from build123d import *

# Parameters (mm, degrees)
SKETCH1_R      = 3.378193244
EXTRUDE1_DEPTH = 300


with BuildPart() as part:
    # Sketch1 → Extrude1 (new body)
    with BuildSketch(Plane.XY):
        with BuildLine():
            Line((-17.04042372, 15.431408639), (-24.485570149, 7.990664768))
            ThreePointArc((-24.485570149, 7.990664768), (-25.653755155, 5.34518984), (-24.733349861, 2.603648687))
            ThreePointArc((-24.733349861, 2.603648687), (-18.529607307, -7.672004621), (-15.653778055, -19.325548231))
            ThreePointArc((-15.653778055, -19.325548231), (-14.366806417, -21.915316136), (-11.67045068, -22.960715361))
            Line((-11.67045068, -22.960715361), (-1.144536244, -22.960715361))
            ThreePointArc((-1.144536244, -22.960715361), (-0.031123661, -22.499524769), (0.430066931, -21.386112187))
            Line((0.430066931, -21.386112187), (0.430066931, -20.471826472))
            ThreePointArc((0.430066931, -20.471826472), (-0.031123661, -19.35841389), (-1.144536244, -18.897223298))
            Line((-1.144536244, -18.897223298), (-1.851013704, -18.897223298))
            ThreePointArc((-1.851013704, -18.897223298), (-2.114950893, -19.003860844), (-2.230734754, -19.263915653))
            Line((-2.230734754, -19.263915653), (-2.231730696, -19.292435705))
            ThreePointArc((-2.231730696, -19.292435705), (-2.347514556, -19.552490514), (-2.611451745, -19.65912806))
            Line((-2.611451745, -19.65912806), (-4.522314022, -19.65912806))
            ThreePointArc((-4.522314022, -19.65912806), (-5.420227395, -19.287200163), (-5.792155291, -18.38928679))
            Line((-5.792155291, -18.38928679), (-5.792155291, -15.94919425))
            ThreePointArc((-5.792155291, -15.94919425), (-5.724492654, -15.609031199), (-5.531805764, -15.320654889))
            Line((-5.531805764, -15.320654889), (-2.245416253, -12.034265378))
            ThreePointArc((-2.245416253, -12.034265378), (-0.704662825, -11.004766851), (1.112779762, -10.643255044))
            Line((1.112779762, -10.643255044), (7.874338227, -10.643255044))
            ThreePointArc((7.874338227, -10.643255044), (9.691780814, -11.004766851), (11.232534242, -12.034265378))
            Line((11.232534242, -12.034265378), (14.518923752, -15.320654889))
            ThreePointArc((14.518923752, -15.320654889), (14.711610642, -15.609031199), (14.77927328, -15.94919425))
            Line((14.77927328, -15.94919425), (14.77927328, -18.38928679))
            ThreePointArc((14.77927328, -18.38928679), (14.407345383, -19.287200163), (13.50943201, -19.65912806))
            Line((13.50943201, -19.65912806), (11.598569733, -19.65912806))
            ThreePointArc((11.598569733, -19.65912806), (11.334632545, -19.552490514), (11.218848684, -19.292435705))
            Line((11.218848684, -19.292435705), (11.217852742, -19.263915653))
            ThreePointArc((11.217852742, -19.263915653), (11.102068882, -19.003860844), (10.838131693, -18.897223298))
            Line((10.838131693, -18.897223298), (10.068162169, -18.897223298))
            ThreePointArc((10.068162169, -18.897223298), (8.994767984, -19.373315236), (8.557051058, -20.462921818))
            Line((8.557051058, -20.462921818), (8.557051058, -21.377207532))
            ThreePointArc((8.557051058, -21.377207532), (8.99769069, -22.469479665), (10.068162169, -22.960715361))
            Line((10.068162169, -22.960715361), (20.406917219, -22.960715361))
            ThreePointArc((20.406917219, -22.960715361), (23.309060919, -21.713452534), (24.401336641, -18.749496331))
            ThreePointArc((24.401336641, -18.749496331), (18.427837191, 7.629867689), (4.005478547, 30.511063307))
            ThreePointArc((4.005478547, 30.511063307), (1.137680997, 31.835389487), (-1.796738453, 30.666079815))
            Line((-1.796738453, 30.666079815), (-9.109504077, 23.357638469))
            ThreePointArc((-9.109504077, 23.357638469), (-9.519412208, 22.253465918), (-9.058959046, 21.169397386))
            Line((-9.058959046, 21.169397386), (-8.412652649, 20.522708582))
            ThreePointArc((-8.412652649, 20.522708582), (-7.332808217, 20.061433598), (-6.237031206, 20.483466005))
            Line((-6.237031206, 20.483466005), (-5.692419534, 21.027755629))
            ThreePointArc((-5.692419534, 21.027755629), (-5.581114397, 21.28975863), (-5.683050759, 21.555546861))
            Line((-5.683050759, 21.555546861), (-5.702507071, 21.576423576))
            ThreePointArc((-5.702507071, 21.576423576), (-5.804443433, 21.842211807), (-5.693138296, 22.104214808))
            Line((-5.693138296, 22.104214808), (-4.341555064, 23.454998805))
            ThreePointArc((-4.341555064, 23.454998805), (-3.443531731, 23.826661124), (-2.545728396, 23.454467682))
            Line((-2.545728396, 23.454467682), (-0.820832785, 21.728551481))
            ThreePointArc((-0.820832785, 21.728551481), (-0.628231192, 21.440118195), (-0.560669162, 21.099935148))
            Line((-0.560669162, 21.099935148), (-0.562043724, 16.452278734))
            ThreePointArc((-0.562043724, 16.452278734), (-0.924093031, 14.634943145), (-1.954047197, 13.094494262))
            Line((-1.954047197, 13.094494262), (-6.736604871, 8.314764671))
            ThreePointArc((-6.736604871, 8.314764671), (-8.27766271, 7.285721873), (-10.095212136, 6.924747597))
            Line((-10.095212136, 6.924747597), (-14.74286855, 6.926122159))
            ThreePointArc((-14.74286855, 6.926122159), (-15.083011574, 6.993885398), (-15.371330884, 7.186657568))
            Line((-15.371330884, 7.186657568), (-17.096226495, 8.91257377))
            ThreePointArc((-17.096226495, 8.91257377), (-17.467888814, 9.810597103), (-17.095695372, 10.708400437))
            Line((-17.095695372, 10.708400437), (-15.74411214, 12.059184434))
            ThreePointArc((-15.74411214, 12.059184434), (-15.482043347, 12.170334575), (-15.216315459, 12.068241015))
            Line((-15.216315459, 12.068241015), (-15.195450256, 12.048772358))
            ThreePointArc((-15.195450256, 12.048772358), (-14.929722367, 11.946678798), (-14.667653575, 12.057828939))
            Line((-14.667653575, 12.057828939), (-14.167950848, 12.557236175))
            ThreePointArc((-14.167950848, 12.557236175), (-13.70643098, 13.67051231), (-14.167292256, 14.784061242))
            Line((-14.167292256, 14.784061242), (-14.813598652, 15.430750047))
            ThreePointArc((-14.813598652, 15.430750047), (-15.926874787, 15.892269915), (-17.04042372, 15.431408639))
        make_face()
        Circle(SKETCH1_R, mode=Mode.SUBTRACT)
        with BuildLine():
            Line((-8.130757209, -21.370715361), (-11.673344577, -21.370715361))
            ThreePointArc((-11.673344577, -21.370715361), (-13.258626812, -20.755471896), (-14.013837102, -19.23189003))
            ThreePointArc((-14.013837102, -19.23189003), (-14.872264525, -13.783171952), (-16.443322189, -8.495714704))
            ThreePointArc((-16.443322189, -8.495714704), (-16.427294419, -7.927487377), (-16.021576747, -7.529326159))
            Line((-16.021576747, -7.529326159), (-6.607938261, -3.630069426))
            ThreePointArc((-6.607938261, -3.630069426), (-6.179406749, -3.609440138), (-5.835565156, -3.866028881))
            ThreePointArc((-5.835565156, -3.866028881), (-4.011915729, -5.736247221), (-1.629593619, -6.807673952))
            ThreePointArc((-1.629593619, -6.807673952), (-1.166319275, -7.252659472), (-1.328408234, -7.874240038))
            Line((-1.328408234, -7.874240038), (-7.148158363, -13.693990167))
            ThreePointArc((-7.148158363, -13.693990167), (-7.312905654, -13.940551912), (-7.370757209, -14.23139132))
            Line((-7.370757209, -14.23139132), (-7.370757209, -20.610715361))
            ThreePointArc((-7.370757209, -20.610715361), (-7.593356055, -21.148116515), (-8.130757209, -21.370715361))
        make_face(mode=Mode.SUBTRACT)
        with BuildLine():
            Line((20.418391526, -21.370715361), (17.138195039, -21.370715361))
            ThreePointArc((17.138195039, -21.370715361), (16.600793885, -21.148116515), (16.378195039, -20.610715361))
            Line((16.378195039, -20.610715361), (16.378195039, -14.25171132))
            ThreePointArc((16.378195039, -14.25171132), (16.320343484, -13.960871912), (16.155596193, -13.714310167))
            Line((16.155596193, -13.714310167), (12.486038977, -10.044752951))
            ThreePointArc((12.486038977, -10.044752951), (10.615478832, -8.794884621), (8.409002698, -8.35598923))
            Line((8.409002698, -8.35598923), (6.154378538, -8.35598923))
            ThreePointArc((6.154378538, -8.35598923), (5.800842447, -8.268753652), (5.528466848, -8.027073394))
            Line((5.528466848, -8.027073394), (4.315683522, -6.266169144))
            ThreePointArc((4.315683522, -6.266169144), (4.209920366, -5.81697222), (4.436221584, -5.414788829))
            ThreePointArc((4.436221584, -5.414788829), (6.594459284, -2.348000586), (6.860062932, 1.392672456))
            ThreePointArc((6.860062932, 1.392672456), (6.921760014, 1.817240818), (7.239364661, 2.105671246))
            Line((7.239364661, 2.105671246), (16.508429277, 5.945043521))
            ThreePointArc((16.508429277, 5.945043521), (17.097304243, 5.94201939), (17.507242876, 5.519250909))
            ThreePointArc((17.507242876, 5.519250909), (21.115407947, -6.478770082), (22.765211001, -18.898492815))
            ThreePointArc((22.765211001, -18.898492815), (22.122756948, -20.638627135), (20.418391526, -21.370715361))
        make_face(mode=Mode.SUBTRACT)
        with BuildLine():
            Line((-19.787590021, 9.363765211), (-15.275025713, 4.851200903))
            ThreePointArc((-15.275025713, 4.851200903), (-15.028463968, 4.686453612), (-14.73762456, 4.628602057))
            Line((-14.73762456, 4.628602057), (-6.507254998, 4.628602057))
            ThreePointArc((-6.507254998, 4.628602057), (-5.953116962, 4.303692426), (-5.966049114, 3.661455717))
            ThreePointArc((-5.966049114, 3.661455717), (-6.933511551, 0.962505882), (-6.737797651, -1.897915388))
            Line((-6.737797651, -1.897915388), (-16.652389322, -6.004673724))
            ThreePointArc((-16.652389322, -6.004673724), (-17.220965814, -6.009958748), (-17.634081109, -5.619263328))
            ThreePointArc((-17.634081109, -5.619263328), (-20.26130976, -0.76628586), (-23.507186823, 3.696673112))
            ThreePointArc((-23.507186823, 3.696673112), (-24.050030989, 5.308183117), (-23.363649832, 6.86398683))
            Line((-23.363649832, 6.86398683), (-20.862233366, 9.363924126))
            ThreePointArc((-20.862233366, 9.363924126), (-20.324878788, 9.586364049), (-19.787590021, 9.363765211))
        make_face(mode=Mode.SUBTRACT)
        with BuildLine():
            Line((-2.989101394, 27.22648713), (-0.664655277, 29.549558726))
            ThreePointArc((-0.664655277, 29.549558726), (1.058380877, 30.23655296), (2.742895641, 29.459877564))
            ThreePointArc((2.742895641, 29.459877564), (10.354016898, 19.511168226), (16.282595001, 8.47676992))
            ThreePointArc((16.282595001, 8.47676992), (16.291564751, 7.888035719), (15.877338122, 7.469580564))
            Line((15.877338122, 7.469580564), (6.607938261, 3.630069426))
            ThreePointArc((6.607938261, 3.630069426), (6.179406749, 3.609440138), (5.835565156, 3.866028881))
            ThreePointArc((5.835565156, 3.866028881), (3.002699742, 6.323274014), (-0.691951535, 6.965716264))
            ThreePointArc((-0.691951535, 6.965716264), (-1.136357264, 7.090083742), (-1.37920161, 7.482499777))
            Line((-1.37920161, 7.482499777), (-1.766781632, 9.585214428))
            ThreePointArc((-1.766781632, 9.585214428), (-1.745076748, 9.94870681), (-1.55677385, 10.260379446))
            Line((-1.55677385, 10.260379446), (0.037486183, 11.854639479))
            ThreePointArc((0.037486183, 11.854639479), (1.287354512, 13.725199623), (1.726249904, 15.931675758))
            Line((1.726249904, 15.931675758), (1.726249904, 21.12121334))
            ThreePointArc((1.726249904, 21.12121334), (1.668398349, 21.412052749), (1.503651058, 21.658614494))
            Line((1.503651058, 21.658614494), (-2.989260356, 26.151525907))
            ThreePointArc((-2.989260356, 26.151525907), (-3.211859194, 26.689039448), (-2.989101394, 27.22648713))
        make_face(mode=Mode.SUBTRACT)
    extrude(amount=-EXTRUDE1_DEPTH)


solid = part.part
The listing builds one solid part. Answer for the finished solid, in the listing's coordinates (mm). A direction names the side the tool comes from. Round coordinates to 2 decimals unless told otherwise and drop trailing zeros. Write each question's results on one line, items separated by ' | '. Start each with the question number.
(1) Determine the mould class of faces 1 (the cylindrical face through (-20.22, -0.83, -147.9)), 2 (the cylindrical face through (-25.65, 5.39, -147.9)), 3 (the cylindrical face through (18.57, 7.28, -147.9)) for opening direction X: +X half, -X half, draft (parallel to the pull), parting line (faces both ways), or undercut.
(2) For faces 4 (the flat face through (-5.402, 27.063, -147.9)), 5 (the cylindrical face through (6.576, -2.398, -147.9)), 6 (the flat face through (4, -10.643, -148)), determine the directions among +Z, -Z, +X, -X, +Y, -Y from which every point of the face is accessible in a straight line to the end or side of a thin tool.
(3) The part is cut by section A-A, the plane z = -221. Give the number of separate pieces and of enclosed holes in the cut face, and give its area (3 significant figures).
(4) Each of these flat-tipped pins is pushed along its axis until it touches: P1, Ø8, axis at x = -17, z = -226.5, coming from the +Y side; P2, Ø3.5, axis at x = -11.5, z = -142, coming from the +Y side; P3, Ø8, axis at x = 8.5, z = -52, coming from the +Y side; P4, Ø7, axis at y = -17.5, z = -91, coming from the +X side. Where does it stop, or does it pass through?
(5) Find the intervals of material crossed by line 1 (X direction, y = -18, z = -100); line 2 (Y direction, x = -11, z = -22); line 3 (X direction, y = 28, z = -114.5), in increasing order.
Worked answers:
1) face 1: undercut | face 2: -X half | face 3: +X half
2) face 4: +Z, -Z, -X, +Y | face 5: +Z, -Z | face 6: +Z, -Z, -Y
3) separate pieces: 1 | enclosed holes: 5 | area: 628 mm²
4) P1: stops at y = 15.89 | P2: stops at y = 6.94 | P3: stops at y = 29.96 | P4: stops at x = 24.41
5) line 1: x = -15.8 to -14.14, -7.37 to -5.79, 14.78 to 16.38, 22.71 to 24.36 | line 2: y = -22.96 to -21.37, -5.45 to -3.66, 4.63 to 6.93 | line 3: x = -4.46 to -2.22, 4.03 to 6.17
